Design review of the part built by this model. Coordinates are the model's own, in mm. A direction names the side the tool comes from. Coordinates: 2 decimals unless noted, no trailing zeros. Write each loop counter-clockwise with the first axis right and the second up, starting at its lowest first coordinate (ties: lowest second). Pieces come first, ordered by that corner, then holes.
Q1. Add section A-A, the plane z = -33.25. Give the boundary of the cut face in (x, y).
Q2. Add section B-B, the plane x = -33.25. Give the boundary of the cut face in (y, z), plus the area to 3 significant figures.
Q3. Add section C-C, the plane y = 3.1. Give the number of separate pieces and of enclosed holes in the cut face, plus the area to 3 significant figures.
Q4. Clearance check with flat-ended pins moving along their axes: pin 1 Ø1.2 at (x, y) = (-20.5, 1.5) entering from +Z; pin 2 Ø1.8 at (x, z) = (-2.75, -2.75) entering from -Y. State where each tip first meets the part, or that it passes through.
Q5. The part is to be moulded in two halves that separate along X. For faces 3 (the face through (-17, 2, 0)), 4 (the face through (-30.25, 2, -3)), 5 (the face through (19.5, 2, -18)), say which applies: +X half, -X half, draft (parallel to the pull), parting line (faces both ways), or undercut.
Q6. To check wall thickness, follow probe 1 along Z at (x, y) = (-46, 3); probe 2 along X at (y, z) = (2.4, -2.75). State the ranges of each line that lie inside material, in increasing order.
Q7. Machinability: for faces 1 (the face through (-30.25, 2, -33)), 2 (the face through (-17, 0, -18)), which of the approach directions +Z, -Z, +X, -X, +Y, -Y give a long, thin tool a straight path to every point of the face, cutting with its end or side? Answer none if there is none.
Autodesk Inventor part; units mm, degrees
ref_plane "YZ Plane" through (0, 0, 0) normal (1, 0, 0) x (0, 1, 0)
ref_plane "XZ Plane" through (0, 0, 0) normal (0, 1, 0) x (-1, 0, 0)
ref_plane "XY Plane" through (0, 0, 0) normal (0, 0, 1) x (1, 0, 0)
sketch "Sketch1" plane through (0, 0, 0) normal (0, 1, 0) x (-1, 0, 0)
  line L0 (0, 0) -> (36, 0)
  line L1 (36, 0) -> (36, -36)
  line L2 (36, -36) -> (0, -36)
  line L3 (0, -36) -> (0, 0)
  line L4 (0, 0) -> (18, 0)
  line L5 (18, 0) -> (18, -18)
  line L6 (18, -18) -> (0, -18)
  line L7 (0, -18) -> (0, 0)
  line L8 (18, -18) -> (33.25, -18)
  line L9 (33.25, -18) -> (33.25, -33.25)
  line L10 (33.25, -33.25) -> (18, -33.25)
  line L11 (18, -33.25) -> (18, -18)
  line L12 (33.25, -33.25) -> (2.75, -33.25)
  line L13 (2.75, -33.25) -> (2.75, -2.75)
  line L14 (2.75, -2.75) -> (33.25, -2.75)
  line L15 (33.25, -2.75) -> (33.25, -33.25)
  circle A0 centre (33.25, -2.75) radius 1
  circle A1 centre (33.25, -33.25) radius 1
  circle A2 centre (2.75, -33.25) radius 1
  circle A3 centre (2.75, -2.75) radius 1
  line L16 (18, -18) -> (55.5, -18)
  line L17 (55.5, -18) -> (55.5, 0)
  line L18 (55.5, 0) -> (18, 0)
  line L19 (18, 0) -> (18, -18)
  line L20 (55.5, 0) -> (-19.5, 0)
  line L21 (-19.5, 0) -> (-19.5, -36)
  line L22 (-19.5, -36) -> (55.5, -36)
  line L23 (55.5, -36) -> (55.5, 0)
  line L24 (-19.5, 0) -> (55.5, 0)
  line L25 (55.5, 0) -> (55.5, 10)
  line L26 (55.5, 10) -> (-19.5, 10)
  line L27 (-19.5, 10) -> (-19.5, 0)
  line L28 (-19.5, -36) -> (55.5, -36)
  line L29 (55.5, -36) -> (55.5, -46)
  line L30 (55.5, -46) -> (-19.5, -46)
  line L31 (-19.5, -46) -> (-19.5, -36)
  dimension "d0" = 36
  dimension "d1" = 36
  dimension "d2" = 18
  dimension "d3" = 18
  dimension "d4" = 15.25
  dimension "d5" = 15.25
  dimension "d6" = 30.5
  dimension "d7" = 30.5
  dimension "d8" = 2
  dimension "d9" = 2
  dimension "d10" = 2
  dimension "d11" = 2
  dimension "d12" = 37.5
  dimension "d13" = 75
  dimension "d16" = 75
  dimension "d17" = 10
  dimension "d18" = 75
  dimension "d19" = 10
extrude "Extrusion1" add sketch "Sketch1" along normal blind 4 contours L0 L5 L14 A3 L13 L6 L3 | L3 L22 L21 L20 | L0 L1 L16 L15 A0 L14 L5 | L6 L13 A2 L12 L10 A1 L9 L16 L1 L2 L3 | L18 L17 L16 L1 | L14 A0 L15 L8 L5 | L5 L6 L13 A3 L14 | L6 L11 L12 A2 L13 | L16 L23 L22 L1 | L8 L9 A1 L10 L11
sketch "Sketch2" plane through (0, 4, 0) normal (0, 1, 0) x (1, 0, 0)
  circle A0 centre (-33.25, 2.75) radius 1
  line L0 (-33.25, 3.75) -> (-33.25, 1.75)
  line L1 (-33.25, 3.75) -> (-30.25, 3.75)
  line L2 (-30.25, 3.75) -> (-30.25, 1.75)
  line L3 (-30.25, 1.75) -> (-33.25, 1.75)
  line L4 (-33.25, 1.75) -> (-33.25, 3.75)
  line L5 (-30.25, 1.75) -> (-30.25, 3.75)
  line L6 (-55.5, 0) -> (19.5, 0)
  line L7 (19.5, 0) -> (19.5, 36)
  line L8 (-55.5, 0) -> (19.5, 0)
  line L9 (19.5, 0) -> (19.5, 18)
  line L10 (19.5, 18) -> (-55.5, 18)
  line L11 (-55.5, 18) -> (-55.5, 0)
  line L12 (-33.25, 3.75) -> (-55.5, 3.75)
  line L13 (-55.5, 3.75) -> (-55.5, 1.75)
  line L14 (-55.5, 1.75) -> (-33.25, 1.75)
  line L15 (-33.25, 1.75) -> (-33.25, 3.75)
  line L16 (-33.25, 3.75) -> (-36.25, 3.75)
  line L17 (-36.25, 3.75) -> (-36.25, 1.75)
  line L18 (-36.25, 1.75) -> (-33.25, 1.75)
  line L19 (-33.25, 1.75) -> (-33.25, 3.75)
  line L20 (-55.5, 3.75) -> (-52.5, 3.75)
  line L21 (-52.5, 3.75) -> (-52.5, 1.75)
  line L22 (-52.5, 1.75) -> (-55.5, 1.75)
  line L23 (-55.5, 1.75) -> (-55.5, 3.75)
  line L24 (-55.5, 36) -> (-55.5, 0)
  line L25 (-55.5, 36) -> (-18, 36)
  line L26 (-18, 36) -> (-18, 0)
  line L27 (-18, 0) -> (-55.5, 0)
  line L28 (-55.5, 0) -> (-55.5, 36)
  line L29 (-30.25, 3.75) -> (-18, 3.75)
  line L30 (-18, 3.75) -> (-18, 1.75)
  line L31 (-18, 1.75) -> (-30.25, 1.75)
  line L32 (-30.25, 1.75) -> (-30.25, 3.75)
  circle A1 centre (-33.25, 33.25) radius 1
  line L33 (-33.25, 32.25) -> (-33.25, 34.25)
  line L34 (-33.25, 32.25) -> (-30.25, 32.25)
  line L35 (-30.25, 32.25) -> (-30.25, 34.25)
  line L36 (-30.25, 34.25) -> (-33.25, 34.25)
  line L37 (-33.25, 34.25) -> (-33.25, 32.25)
  line L38 (-30.25, 34.25) -> (-30.25, 32.25)
  line L39 (-33.25, 32.25) -> (-55.5, 32.25)
  line L40 (-55.5, 32.25) -> (-55.5, 34.25)
  line L41 (-55.5, 34.25) -> (-33.25, 34.25)
  line L42 (-33.25, 34.25) -> (-33.25, 32.25)
  line L43 (-33.25, 32.25) -> (-36.25, 32.25)
  line L44 (-36.25, 32.25) -> (-36.25, 34.25)
  line L45 (-36.25, 34.25) -> (-33.25, 34.25)
  line L46 (-33.25, 34.25) -> (-33.25, 32.25)
  line L47 (-55.5, 32.25) -> (-52.5, 32.25)
  line L48 (-52.5, 32.25) -> (-52.5, 34.25)
  line L49 (-52.5, 34.25) -> (-55.5, 34.25)
  line L50 (-55.5, 34.25) -> (-55.5, 32.25)
  line L51 (-30.25, 32.25) -> (-18, 32.25)
  line L52 (-18, 32.25) -> (-18, 34.25)
  line L53 (-18, 34.25) -> (-30.25, 34.25)
  line L54 (-30.25, 34.25) -> (-30.25, 32.25)
  circle A2 centre (-2.75, 2.75) radius 1
  line L55 (-2.75, 3.75) -> (-2.75, 1.75)
  line L56 (-2.75, 3.75) -> (-5.75, 3.75)
  line L57 (-5.75, 3.75) -> (-5.75, 1.75)
  line L58 (-5.75, 1.75) -> (-2.75, 1.75)
  line L59 (-2.75, 1.75) -> (-2.75, 3.75)
  line L60 (-5.75, 1.75) -> (-5.75, 3.75)
  line L61 (19.5, 18) -> (19.5, 0)
  line L62 (-2.75, 3.75) -> (19.5, 3.75)
  line L63 (19.5, 3.75) -> (19.5, 1.75)
  line L64 (19.5, 1.75) -> (-2.75, 1.75)
  line L65 (-2.75, 1.75) -> (-2.75, 3.75)
  line L66 (-2.75, 3.75) -> (0.25, 3.75)
  line L67 (0.25, 3.75) -> (0.25, 1.75)
  line L68 (0.25, 1.75) -> (-2.75, 1.75)
  line L69 (-2.75, 1.75) -> (-2.75, 3.75)
  line L70 (19.5, 3.75) -> (16.5, 3.75)
  line L71 (16.5, 3.75) -> (16.5, 1.75)
  line L72 (16.5, 1.75) -> (19.5, 1.75)
  line L73 (19.5, 1.75) -> (19.5, 3.75)
  line L74 (19.5, 36) -> (19.5, 0)
  line L75 (19.5, 36) -> (-18, 36)
  line L76 (-18, 0) -> (19.5, 0)
  line L77 (19.5, 0) -> (19.5, 36)
  line L78 (-5.75, 3.75) -> (-18, 3.75)
  line L79 (-18, 1.75) -> (-5.75, 1.75)
  line L80 (-5.75, 1.75) -> (-5.75, 3.75)
  circle A3 centre (-2.75, 33.25) radius 1
  line L81 (-2.75, 32.25) -> (-2.75, 34.25)
  line L82 (-2.75, 32.25) -> (19.5, 32.25)
  line L83 (19.5, 34.25) -> (-2.75, 34.25)
  line L84 (16.5, 32.25) -> (16.5, 34.25)
  line L85 (19.5, 32.25) -> (16.5, 32.25)
  line L86 (16.5, 34.25) -> (19.5, 34.25)
  line L87 (19.5, 32.25) -> (19.5, 34.25)
  line L88 (19.5, 34.25) -> (19.5, 32.25)
  line L89 (0.25, 32.25) -> (0.25, 34.25)
  line L90 (-2.75, 32.25) -> (0.25, 32.25)
  line L91 (-2.75, 34.25) -> (-2.75, 32.25)
  line L92 (-2.75, 34.25) -> (-2.75, 32.25)
  line L93 (-2.75, 34.25) -> (-2.75, 32.25)
  line L94 (-2.75, 32.25) -> (-5.75, 32.25)
  line L95 (-5.75, 32.25) -> (-5.75, 34.25)
  line L96 (-5.75, 34.25) -> (-5.75, 32.25)
  line L97 (-5.75, 34.25) -> (-2.75, 34.25)
  line L98 (0.25, 34.25) -> (-2.75, 34.25)
  line L99 (-5.75, 34.25) -> (-5.75, 32.25)
  line L100 (-5.75, 32.25) -> (-18, 32.25)
  line L101 (-18, 34.25) -> (-5.75, 34.25)
  dimension "d20" = 3
  dimension "d24" = 3
  dimension "d25" = 3
extrude "Extrusion2" cut sketch "Sketch2" against normal up to surface (4 mm away) contours L29 L26 L31 L2 | L17 L14 L21 L12 | L78 L57 L79 L26 | L51 L35 L53 L26 | L26 L101 L95 L100 | L62 L71 L64 L67 | L82 L89 L83 L84 | L48 L41 L44 L39
properties part number "base"
Here are the results:
1. outline: (-55.5, 0) - (-52.5, 0) - (-52.5, 4) - (-55.5, 4) - close; (-36.25, 0) - (-34.25, 0) - (-34.25, 4) - (-36.25, 4) - close; (-32.25, 0) - (-30.25, 0) - (-30.25, 4) - (-32.25, 4) - close; (-5.75, 0) - (-3.75, 0) - (-3.75, 4) - (-5.75, 4) - close; (-1.75, 0) - (0.25, 0) - (0.25, 4) - (-1.75, 4) - close; (16.5, 0) - (19.5, 0) - (19.5, 4) - (16.5, 4) - close
2. outline: (0, -36) - (4, -36) - (4, -34.25) - (0, -34.25) - close; (0, -32.25) - (4, -32.25) - (4, -3.75) - (0, -3.75) - close; (0, -1.75) - (4, -1.75) - (4, 0) - (0, 0) - close
2. area: 128 mm2
3. separate pieces: 1
3. enclosed holes: 10
3. area: 2,460 mm2
4. pin 1: stops at z = 0
4. pin 2: passes through
5. face 3: draft
5. face 4: undercut
5. face 5: +X half
6. probe 1: z = -36 to -34.25, -32.25 to -3.75, -1.75 to 0
6. probe 2: x = -55.5 to -52.5, -36.25 to -34.25, -32.25 to -30.25, -5.75 to -3.75, -1.75 to 0.25, 16.5 to 19.5
7. face 1: +Y, -Y
7. face 2: +Z, -Z, +X, -X, -Y
